Input: part model. Units: mm. Frame: model coordinates. A direction names the side the tool comes from. Coordinates: 2 decimals unless noted, no trailing zeros. Order: outer loops, then holes, each group sorted by start corner. A loop starts at its lowest first (then second) coordinate and runs counter-clockwise, first axis right, second up. Notation, with made-up numbers: M 42.25,25 L 92.25,25 A12 ccw 92.25,34 Z; hole C 88.25,-9.75 d2. An arc over 180 degrees is marked long. Answer in a Markdown table with one row per item.
from build123d import *

# Parameters (mm, degrees)
F0_R     = 11.328224
F1_DEPTH = 50.8
F0_R_2   = 15.236447
F2_DEPTH = 12.7
F3_R     = 1.687605
F4_DEPTH = 1.524


with BuildPart() as f1:
    # F0 (on Top) → F1 (new body)
    with BuildSketch(Plane.XY):
        Circle(F0_R)
    extrude(amount=-F1_DEPTH)

    # F0 (on Top) → F2 (join)
    with BuildSketch(Plane.XY):
        Circle(F0_R_2)
        Circle(F0_R, mode=Mode.SUBTRACT)
    extrude(amount=-F2_DEPTH)

    # F3 (on Top) → F4 (join)
    with BuildSketch(Plane.XY):
        Circle(F3_R)
        with BuildLine():
            ThreePointArc((-2.193762, -2.115145), (-3.044929, 0.121791), (-2.017821, 2.2836))
            Line((-2.017821, 2.2836), (-2.92536, 3.240976))
            ThreePointArc((-2.92536, 3.240976), (-4.3603, 0.222363), (-3.239887, -2.926566))
            Line((-3.239887, -2.926566), (-2.193762, -2.115145))
        make_face()
        with BuildLine():
            ThreePointArc((-4.267654, -3.723748), (-5.65473, 0.321247), (-3.818462, 4.183123))
            Line((-3.818462, 4.183123), (-4.804929, 5.223764))
            ThreePointArc((-4.804929, 5.223764), (-7.084475, 0.430437), (-5.402019, -4.603612))
            Line((-5.402019, -4.603612), (-4.267654, -3.723748))
        make_face()
        with BuildLine():
            ThreePointArc((-6.64799, -5.570042), (-8.65553, 0.550403), (-5.888899, 6.367261))
            Line((-5.888899, 6.367261), (-7.230815, 7.782869))
            ThreePointArc((-7.230815, 7.782869), (-10.600437, 0.698907), (-8.19006, -6.76614))
            Line((-8.19006, -6.76614), (-6.64799, -5.570042))
        make_face()
        with BuildLine():
            Line((3.264468, 2.899122), (2.304564, 1.993843))
            ThreePointArc((2.304564, 1.993843), (3.047234, -0.028162), (2.26732, -2.036096))
            Line((2.26732, -2.036096), (3.279597, -2.881997))
            ThreePointArc((3.279597, -2.881997), (4.365951, 0.011425), (3.264468, 2.899122))
        make_face()
        with BuildLine():
            ThreePointArc((4.209008, 3.78991), (5.663624, 0.050381), (4.275763, -3.714434))
            Line((4.275763, -3.714434), (5.376066, -4.633893))
            ThreePointArc((5.376066, -4.633893), (7.096924, 0.093408), (5.252245, 4.77378))
            Line((5.252245, 4.77378), (4.209008, 3.78991))
        make_face()
        with BuildLine():
            ThreePointArc((6.398567, 5.854868), (8.671871, 0.140687), (6.585121, -5.644229))
            Line((6.585121, -5.644229), (8.081886, -6.894988))
            ThreePointArc((8.081886, -6.894988), (10.621584, 0.199216), (7.817651, 7.193196))
            Line((7.817651, 7.193196), (6.398567, 5.854868))
        make_face()
    extrude(amount=F4_DEPTH)


solid = f1.part
1) Cut plane A-A, the plane x = 0. Output: boundary loops of the cut face in (y, z), and give its area (3 significant figures).
Resolved:
| item | result |
|---|---|
| outline | M -15.24,-12.7 L -11.33,-12.7 L -11.33,-50.8 L 11.33,-50.8 L 11.33,-12.7 L 15.24,-12.7 L 15.24,0 L 1.69,0 L 1.69,1.52 L -1.69,1.52 L -1.69,0 L -15.24,0 Z |
| area | 1,260 mm2 |
2) Cut plane D-D, the plane z = -24.5. Output: boundary loops of the cut face in (x, y), and give its area (3 significant figures).
Resolved:
| item | result |
|---|---|
| outline | C 0,0 d22.66 |
| area | 403 mm2 |
3) Material intervals for probe 1 along Z at (x, y) = (5.5, 6); probe 2 along Z at (x, y) = (-12.5, -0.5); probe 3 along Y at (x, z) = (4, -27.5), sorted ascending.
Resolved:
| item | result |
|---|---|
| probe 1 | z = -50.8 to 0 |
| probe 2 | z = -12.7 to 0 |
| probe 3 | y = -10.6 to 10.6 |
4) Reachability of faces 5 (the face through (0, 0, 1.524)), 6 (the face through (-6.55, 7.065, 0.751)), 7 (the face through (0, 0, -50.8)), 8 (the face through (4.82, -4.17, 0.75)), 9 (the face through (7.098, 0.021, 0.751)) from +Z, -Z, +X, -X, +Y, -Y: full face, straight path, thin tool, end or side. Return the list, or none.
Resolved:
| item | result |
|---|---|
| face 5 | +Z, +X, -X, +Y, -Y |
| face 6 | +Z, +Y |
| face 7 | -Z, +X, -X, +Y, -Y |
| face 8 | +Z, -Y |
| face 9 | +Z |
5) Mould query, pull axis X, two halves, no side actions, for faces 1 (the face through (-2.3, 11.4, -12.7)), 2 (the face through (0, -3, 0)), 3 (the face through (-10.592, 0.811, 0.751)), 4 (the face through (4.366, -0.033, 0.751)). Classes: +X half, -X half, draft (parallel to the pull), parting line (faces both ways), or undercut.
Resolved:
| item | result |
|---|---|
| face 1 | draft |
| face 2 | undercut |
| face 3 | -X half |
| face 4 | undercut |
6) Cut plane C-C, the plane z = -7.5. Output: boundary loops of the cut face in (x, y).
Resolved:
| item | result |
|---|---|
| outline | C 0,0 d30.47 |
7) Cut plane B-B, the plane y = -10.5. Output: boundary loops of the cut face in (x, z).
Resolved:
| item | result |
|---|---|
| outline | M -11.04,-12.7 L -4.25,-12.7 L -4.25,-50.8 L 4.25,-50.8 L 4.25,-12.7 L 11.04,-12.7 L 11.04,0 L -11.04,0 Z |
8) Contact query for flat-ended pins moving along their axis: pin 1 (4 mm diameter, centred on y = -2, z = -34, fed in from +X); pin 2 (3 mm diameter, centred on x = -11.5, z = -26, fed in from -Y); pin 3 (5 mm diameter, centred on x = -6.5, z = -14.5, fed in from -Y); pin 4 (10 mm diameter, centred on x = -6, y = -11, fed in from -Z). Output: stop coordinate, or through.
Resolved:
| item | result |
|---|---|
| pin 1 | stops at x = 11.33 |
| pin 2 | stops at y = -5.32 |
| pin 3 | stops at y = -14.47 |
| pin 4 | stops at z = -50.8 |
